```python
from build123d import *


with BuildPart() as f1:
    # F0 (on Front) → F1 (revolve)
    with BuildSketch(Plane.XZ):
        with BuildLine():
            Line((-100, 0), (0, 0))
            Line((0, 0), (0, 3.010338))
            ThreePointArc((0, 3.010338), (-0.659512, 4.494619), (-2.203091, 5))
            Line((-2.203091, 5), (-12, 4))
            Line((-12, 4), (-20, 4))
            Line((-20, 4), (-30, 6.5))
            Line((-30, 6.5), (-40, 6.5))
            Line((-40, 6.5), (-50, 5))
            Line((-50, 5), (-60, 9.5))
            Line((-60, 9.5), (-100, 9.5))
            Line((-100, 9.5), (-100, 0))
        make_face()
    revolve(axis=Axis((-50, 0, 0), (1, 0, 0)))


solid = f1.part
```
Check sheet for the modelled part. Datum: model origin and axes. Units: mm. A direction names the side the tool comes from. Give positions to 0.01 mm unless a question says otherwise; leave off trailing zeros. Write each loop counter-clockwise with the first axis right and the second up, starting at its lowest first coordinate (ties: lowest second). Pieces come first, ordered by that corner, then holes.
Item 1: Cross-section at A-A (y = 0). Enter the section's corners in (x, z), and give its area (3 significant figures).
Item 2: Draft check along X on faces 1 (the face through (-80.28, 8.43, 4.38)), 2 (the face through (-100, 0, 0)), 3 (the face through (-23.959, -4.947, -0.65)), 4 (the face through (-46.181, 4.944, 2.572)). Enter one of: released by +X, released by -X, zero draft, split by the parting line, or undercut.
Item 3: Gauge pin test, flat ends, axial feed: pin 1 (10 mm diameter, centred on y = -4, z = -6.5, fed in from +X); pin 2 (6 mm diameter, centred on x = -25, y = -1, fed in from -Z); pin 3 (6 mm diameter, centred on x = -85, z = 7, fed in from -Y); pin 4 (6 mm diameter, centred on x = -75, z = 4.5, fed in from +Y). Record the tip position at first contact, or that the pin passes through.
Item 4: Access from +Z, -Z, +X, -X, +Y, -Y to the whole of each face (thin tool, end or side, straight path). Record for faces 5 (the face through (-35.07, 3.955, -5.158)), 6 (the face through (0, 0, 0)), 7 (the face through (-52.85, -1.89, 5.99)).
Item 5: Scan lines: L1, parallel to Y at x = -90, z = 0.25; L2, parallel to Y at x = -19.5, z = 3.25; L3, parallel to Z at x = -69, y = 6. Record each from-to range of solid material in increasing order.
Report:
1. outline: (-100, -9.5) - (-60, -9.5) - (-50, -5) - (-40, -6.5) - (-30, -6.5) - (-20, -4) - (-12, -4) - (-2.2, -5) arc R2 ccw to (0, -3.01) - (0, 3.01) arc R2 ccw to (-2.2, 5) - (-12, 4) - (-20, 4) - (-30, 6.5) - (-40, 6.5) - (-50, 5) - (-60, 9.5) - (-100, 9.5) - close
1. area: 1,430 mm2
2. face 1: zero draft
2. face 2: released by -X
2. face 3: undercut
2. face 4: undercut
3. pin 1: stops at x = 0
3. pin 2: stops at z = -5.97
3. pin 3: stops at y = -8.62
3. pin 4: stops at y = 9.38
4. face 5: +X
4. face 6: +Z, -Z, +X, +Y, -Y
4. face 7: none
5. L1: y = -9.5 to 9.5
5. L2: y = -2.33 to 2.33
5. L3: z = -7.37 to 7.37
